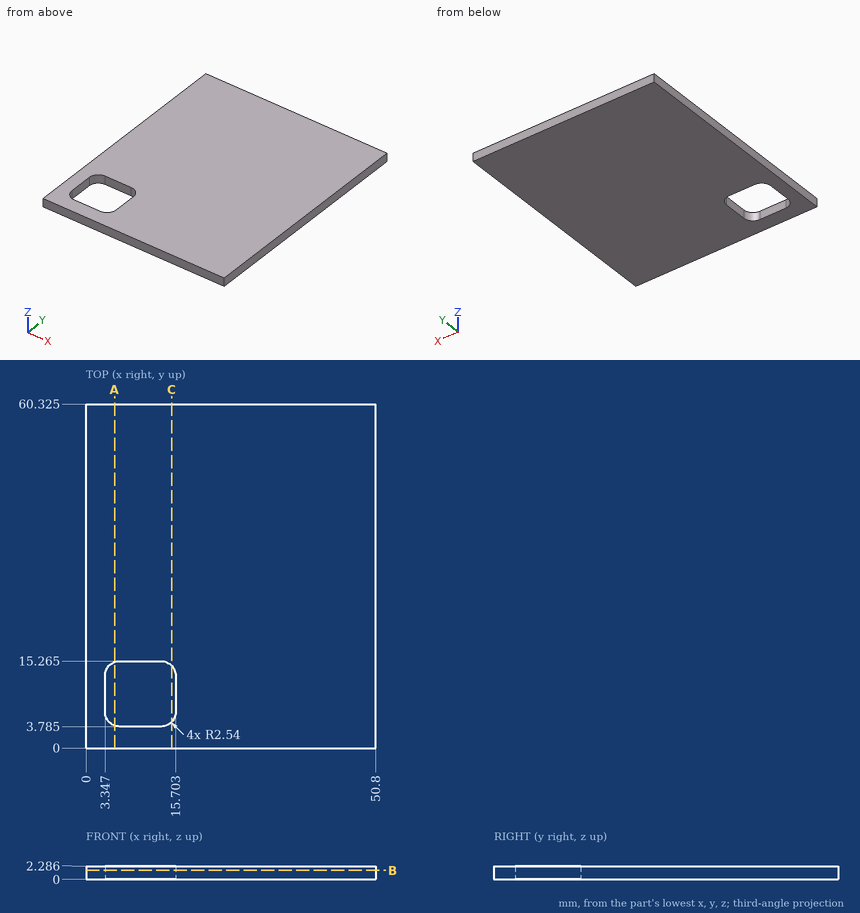
Geometry check sheet. Reference: drawing and pictorial views, mm from the part's lowest x, y, z. Give positions to 0.01 mm unless a question says otherwise; leave off trailing zeros. Order: outer loops, then holes, each group sorted by start corner. A loop starts at its lowest first (then second) coordinate and runs counter-clockwise, first axis right, second up. Notation, with made-up numbers: M -0.75,52.5 L 39.25,52.5 A19 ccw 39.25,65.5 Z; hole C -19.5,-31.5 d7. An arc over 180 degrees is marked long. Answer in a Markdown table with one row per item.
1) Cross-section at B-B, the plane z = 1.55. Enter the section's corners in (x, y) (1 decimal), plus the area to 3 significant figures.
Filled sheet:
| item | result |
|---|---|
| outline | M 0,0 L 50.8,0 L 50.8,60.3 L 0,60.3 Z; hole M 3.3,6.3 A2.5 ccw 5.9,3.8 L 13.2,3.8 A2.5 ccw 15.7,6.3 L 15.7,12.7 A2.5 ccw 13.2,15.3 L 5.9,15.3 A2.5 ccw 3.3,12.7 Z |
| area | 2,930 mm2 |
2) Thickness scan on L1, parallel to Y at x = 6, z = 1.5 (1 decimal); L2, parallel to X at y = 13, z = 1.8; L3, parallel to X at y = 4, z = 0.7 (1 decimal). Record the ranges inside material, lowest first. Write a range as [from, to].
Filled sheet:
| item | result |
|---|---|
| L1 | y = [0, 3.8], [15.3, 60.3] |
| L2 | x = [0, 3.36], [15.69, 50.8] |
| L3 | x = [0, 4.9], [14.2, 50.8] |
3) Cross-section at C-C, the plane x = 15. Enter the section's corners in (y, z) (3 decimals).
Filled sheet:
| item | result |
|---|---|
| outline | M 0,0 L 4.571,0 L 4.571,2.286 L 0,2.286 Z; M 14.479,0 L 60.325,0 L 60.325,2.286 L 14.479,2.286 Z |
4) Cross-section at A-A, the plane x = 5. Enter the section's corners in (y, z) (3 decimals).
Filled sheet:
| item | result |
|---|---|
| outline | M 0,0 L 3.945,0 L 3.945,2.286 L 0,2.286 Z; M 15.105,0 L 60.325,0 L 60.325,2.286 L 15.105,2.286 Z |
